Design review of the part built by this model. Coordinates are the model's own, in mm. A direction names the side the tool comes from. Give positions to 0.01 mm unless a question says otherwise; leave off trailing zeros. Write each loop counter-clockwise with the first axis right and the second up, starting at its lowest first coordinate (ties: lowest second). Pieces come first, ordered by that corner, then holes. Notation, with made-up numbers: M 34.5,85 L 63.5,85 A24 ccw 63.5,113 Z; hole C -26,-25.5 d5. An arc over 180 degrees is marked long. Answer in a Markdown table with one row per item.
```python
from build123d import *

# Parameters (mm, degrees)
SKETCH1_R           = 60
BOSS_EXTRUDE1_DEPTH = 10
SKETCH2_R           = 4.92
BOSS_EXTRUDE2_DEPTH = 30
CIRPATTERN1_COUNT   = 2


with BuildPart() as part:
    # Sketch1 → Boss-Extrude1 (new body)
    with BuildSketch(Plane.XY):
        Circle(SKETCH1_R)
    extrude(amount=BOSS_EXTRUDE1_DEPTH)

    # Sketch2 → Boss-Extrude2 (add)
    with BuildSketch(Plane.XY):
        with Locations((0, 45.984931592)):
            Circle(SKETCH2_R)
    boss_extrude2 = extrude(amount=BOSS_EXTRUDE2_DEPTH)

    # CirPattern1: Boss-Extrude2 ×2 about axis
    cirpattern1_axis = Axis((0, 0, 0), (0, 0, 1))
    for i in range(1, CIRPATTERN1_COUNT):
        add(boss_extrude2.rotate(cirpattern1_axis, i * 360 / CIRPATTERN1_COUNT))


solid = part.part
```
1) The part is to be moulded in two halves that separate along Y. For faces 1 (the face through (-59.94, 2.64, 4.93)), 2 (the face through (1.067, -41.182, 19.86)), 3 (the face through (0, 46, 30)), say which applies: released by +Y, released by -Y, zero draft, split by the parting line, or undercut.
Geometry says:
| item | result |
|---|---|
| face 1 | split by the parting line |
| face 2 | undercut |
| face 3 | zero draft |
2) To check wall thickness, follow probe 1 along Z at (x, y) = (-13.5, -10.5); probe 2 along Y at (x, z) = (-3, 25.5); probe 3 along X at (y, z) = (-3, 6). State the ranges of each line that lie inside material, in increasing order. Write a range as [from, to].
Geometry says:
| item | result |
|---|---|
| probe 1 | [0, 10] |
| probe 2 | [-49.88, -42.09], [42.09, 49.88] |
| probe 3 | [-59.92, 59.92] |
3) Add section B-B (y = 0). Write out the cut boundary in (x, z), and give its area (3 significant figures).
Geometry says:
| item | result |
|---|---|
| outline | M -60,0 L 60,0 L 60,10 L -60,10 Z |
| area | 1,200 mm^2 |
4) For faces 4 (the face through (0, -46, 30)), 5 (the face through (-1.067, 41.182, 19.86)), list the 3-axis set-ups (+Z, -Z, +X, -X, +Y, -Y) from which the entire face can be reached by the end or side of a thin tool; tool diameter is ignored.
Geometry says:
| item | result |
|---|---|
| face 4 | +Z, +X, -X, +Y, -Y |
| face 5 | +Z |
5) Add section A-A (x = 0). Write out the cut boundary in (y, z).
Geometry says:
| item | result |
|---|---|
| outline | M -60,0 L 60,0 L 60,10 L 50.9,10 L 50.9,30 L 41.06,30 L 41.06,10 L -41.06,10 L -41.06,30 L -50.9,30 L -50.9,10 L -60,10 Z |
6) Insertion check: P1, Ø1, axis at x = 6, y = -23, coming from the +Z side; P2, Ø5, axis at y = 16, z = 5.5, coming from the +X side. Each pin has a flat end and moves straight along its axis. Give the tip position at first contact, or say it passes through.
Geometry says:
| item | result |
|---|---|
| P1 | z = 10 |
| P2 | x = 58.46 |
7) Add section C-C (z = 24.75). Write out the cut boundary in (x, y).
Geometry says:
| item | result |
|---|---|
| outline | C 0,-45.98 d9.84; C 0,45.98 d9.84 |
8) Add section D-D (z = 5.25). Write out the cut boundary in (x, y), and give its area (3 significant figures).
Geometry says:
| item | result |
|---|---|
| outline | C 0,0 d120 |
| area | 11,300 mm^2 |
